Geometry check sheet. Reference: the model listing, model coordinates, mm. Face numbers are marked on the shaded views. Give positions to 0.01 mm unless a question says otherwise; leave off trailing zeros.
1. Release check for a two-part mould opening along X. For the marked faces 1, 2 and 3 record: +X half, -X half, draft (parallel to the pull), parting line (faces both ways), or undercut.
2. Material ranges on L1, parallel to Z at x = -225, y = 1159, recorded low to high.
3. Go/stop test with a flat-tipped pin: pin 1 Ø2 at (x, y) = (291.5, 1280.5) entering from +Z. Record where the tip stops, or that it passes through.
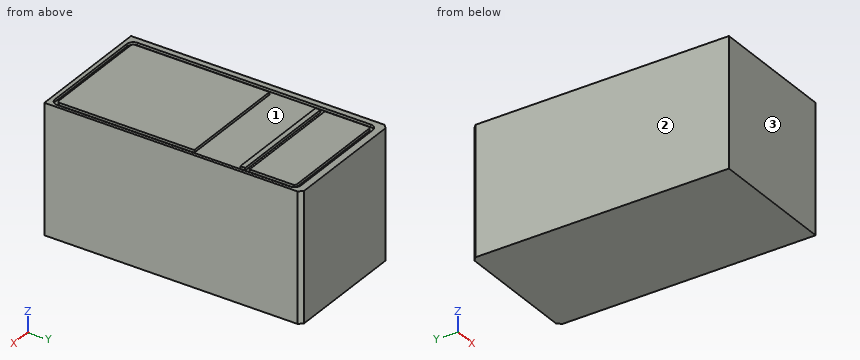
from build123d import *

# Parameters (mm, degrees)
CROQUIS1_W              = 1000
CROQUIS1_H              = 1000
SALIENTE_EXTRUIR1_DEPTH = 2000
CORTAR_EXTRUIR1_DEPTH   = 20
CROQUIS3_W              = 869.3440362
CROQUIS3_H              = 33.772787811
CORTAR_EXTRUIR2_DEPTH   = 20
CHAFL_N1_SIZE           = 30


with BuildPart() as part:
    # Croquis1 → Saliente-Extruir1 (new body)
    with BuildSketch(Plane(origin=(0, 0, 0), x_dir=(1, 0, 0), z_dir=(0, 1, 0))):
        Rectangle(CROQUIS1_W, CROQUIS1_H)
    extrude(amount=SALIENTE_EXTRUIR1_DEPTH)

    # Croquis2 → Cortar-Extruir1 (cut)
    with BuildSketch(Plane.XY.offset(500)):
        with BuildLine():
            Line((-453.105485689, 1895.512731964), (-453.105485689, 82.602501534))
            ThreePointArc((-453.105485689, 82.602501534), (-438.460824748, 47.247162475), (-403.105485689, 32.602501534))
            Line((-403.105485689, 32.602501534), (426.238550511, 32.602501534))
            ThreePointArc((426.238550511, 32.602501534), (461.59388957, 47.247162475), (476.238550511, 82.602501534))
            Line((476.238550511, 82.602501534), (476.238550511, 1895.512731964))
            ThreePointArc((476.238550511, 1895.512731964), (461.59388957, 1930.868071024), (426.238550511, 1945.512731964))
            Line((426.238550511, 1945.512731964), (-403.105485689, 1945.512731964))
            ThreePointArc((-403.105485689, 1945.512731964), (-438.460824748, 1930.868071024), (-453.105485689, 1895.512731964))
        make_face()
        with BuildLine():
            Line((-403.105485689, 1915.512731964), (426.238550511, 1915.512731964))
            ThreePointArc((426.238550511, 1915.512731964), (440.380686134, 1909.654867588), (446.238550511, 1895.512731964))
            Line((446.238550511, 1895.512731964), (446.238550511, 1487.15617354))
            Line((446.238550511, 1487.15617354), (-423.105485689, 1487.15617354))
            Line((-423.105485689, 1487.15617354), (-423.105485689, 1895.512731964))
            ThreePointArc((-423.105485689, 1895.512731964), (-417.247621312, 1909.654867588), (-403.105485689, 1915.512731964))
        make_face(mode=Mode.SUBTRACT)
        with BuildLine():
            Line((-403.105485689, 62.602501534), (426.238550511, 62.602501534))
            ThreePointArc((426.238550511, 62.602501534), (440.380686134, 68.460365911), (446.238550511, 82.602501534))
            Line((446.238550511, 82.602501534), (446.238550511, 1129.448445192))
            Line((446.238550511, 1129.448445192), (-423.105485689, 1129.448445192))
            Line((-423.105485689, 1129.448445192), (-423.105485689, 82.602501534))
            ThreePointArc((-423.105485689, 82.602501534), (-417.247621312, 68.460365911), (-403.105485689, 62.602501534))
        make_face(mode=Mode.SUBTRACT)
    extrude(amount=-CORTAR_EXTRUIR1_DEPTH, mode=Mode.SUBTRACT)

    # Croquis3 → Cortar-Extruir2 (cut)
    with BuildSketch(Plane.XY.offset(500)):
        with Locations((11.566532411, 1542.475404205)):
            Rectangle(CROQUIS3_W, CROQUIS3_H)
    extrude(amount=-CORTAR_EXTRUIR2_DEPTH, mode=Mode.SUBTRACT)

    # Chaflán1
    chafl_n1_edges = [part.edges().sort_by_distance(p)[0] for p in [
        (-500, 2000, 0),
        (500, 2000, 0),
    ]]
    chamfer(chafl_n1_edges, length=CHAFL_N1_SIZE)


solid = part.part
Result:
1. face 1: undercut
1. face 2: -X half
1. face 3: draft
2. L1: z = -500 to 480
3. pin 1: stops at z = 480
